```python
from build123d import *

# Parameters (mm, degrees)
BOSS_EXTRUDE2_DEPTH   = 22
SKETCH6_R             = 6
BOSS_EXTRUDE3_DEPTH   = 8
BOSS_EXTRUDE4_DEPTH   = 65
SKETCH8_R             = 3
CUT_EXTRUDE5_DEPTH    = 65
SKETCH9_R             = 6
CUT_EXTRUDE6_DEPTH    = 52
M4_TAPPED_HOLE1_D     = 3.3
M4_TAPPED_HOLE1_DEPTH = 14
M4_TAPPED_HOLE1_TIP   = 0.991420021
SKETCH13_R            = 1.5
SKETCH13_R_2          = 2.5
CUT_EXTRUDE7_DEPTH    = 5
SKETCH14_R            = 1
CUT_EXTRUDE8_DEPTH    = 15
CHAMFER1_SIZE         = 1


with BuildPart() as part:
    # Sketch2 → Boss-Extrude2 (new body)
    with BuildSketch(Plane(origin=(0, 0, 0), x_dir=(1, 0, 0), z_dir=(0, 1, 0))):
        with BuildLine():
            Line((3.31662479, -5), (-3.31662479, -5))
            ThreePointArc((-3.31662479, -5), (0, 6), (3.31662479, -5))
        make_face()
    extrude(amount=BOSS_EXTRUDE2_DEPTH)

    # Sketch6 → Boss-Extrude3 (add)
    with BuildSketch(Plane(origin=(0, 22, 0), x_dir=(1, 0, 0), z_dir=(0, 1, 0))):
        with Locations(Location((0, 0, 0), (0, 0, 236.442690238))):
            Circle(SKETCH6_R)
    extrude(amount=BOSS_EXTRUDE3_DEPTH)

    # Sketch7 → Boss-Extrude4 (add)
    with BuildSketch(Plane(origin=(0, 30, 0), x_dir=(1, 0, 0), z_dir=(0, 1, 0))):
        with BuildLine():
            Line((-13, 5.196152423), (-13, -5.196152423))
            ThreePointArc((-13, -5.196152423), (14, 0), (-13, 5.196152423))
        make_face()
    extrude(amount=BOSS_EXTRUDE4_DEPTH)

    # Sketch8 → Cut-Extrude5 (cut)
    with BuildSketch(Plane(origin=(0, 95, 0), x_dir=(1, 0, 0), z_dir=(0, 1, 0))):
        with Locations(Location((-8, 0, 0), (0, 0, 270))):
            Circle(SKETCH8_R)
    extrude(amount=-CUT_EXTRUDE5_DEPTH, mode=Mode.SUBTRACT)

    # Sketch9 → Cut-Extrude6 (cut)
    with BuildSketch(Plane(origin=(0, 95, 0), x_dir=(1, 0, 0), z_dir=(0, 1, 0))):
        with Locations(Location((5, 0, 0), (0, 0, 270))):
            Circle(SKETCH9_R)
    extrude(amount=-CUT_EXTRUDE6_DEPTH, mode=Mode.SUBTRACT)

    # M4 Tapped Hole1
    with Locations(Plane(origin=(0, 95, -9), x_dir=(0, 0, 1), z_dir=(0, 1, 0))):
        with Locations((0, 0), (18, 0)):
            Hole(M4_TAPPED_HOLE1_D / 2, depth=M4_TAPPED_HOLE1_DEPTH)
            with Locations((0, 0, -(M4_TAPPED_HOLE1_DEPTH + M4_TAPPED_HOLE1_TIP / 2))):  # 118° drill point
                Cone(0, M4_TAPPED_HOLE1_D / 2, M4_TAPPED_HOLE1_TIP, mode=Mode.SUBTRACT)

    # Sketch13 → Cut-Extrude7 (cut)
    with BuildSketch(Plane.ZY.offset(13)):
        with Locations((0, 34)):
            Circle(SKETCH13_R)
        with Locations((0, 63)):
            Circle(SKETCH13_R_2)
    extrude(amount=-CUT_EXTRUDE7_DEPTH, mode=Mode.SUBTRACT)

    # Sketch14 → Cut-Extrude8 (cut)
    with BuildSketch(Plane.ZY.offset(13)):
        with Locations((0, 85)):
            Circle(SKETCH14_R)
        with Locations((0, 43)):
            Circle(SKETCH14_R)
    extrude(amount=-CUT_EXTRUDE8_DEPTH, mode=Mode.SUBTRACT)

    # Chamfer1
    chamfer1_edges = [part.edges().sort_by_distance(p)[0] for p in [
        (0, 0, 5),
        (0, 0, -6),
    ]]
    chamfer(chamfer1_edges, length=CHAMFER1_SIZE - 0.0001)  # a hair under: the kernel refuses the full size


solid = part.part
```
Model file for the job. Use its own axes, mm. A direction names the side the tool comes from. Coordinates: 2 decimals unless noted, no trailing zeros. Order: outer loops, then holes, each group sorted by start corner. A loop starts at its lowest first (then second) coordinate and runs counter-clockwise, first axis right, second up. Notation, with made-up numbers: (-35.5, 28) - (11.5, 28) arc R7 ccw to (11.5, 39) - close; hole circle Ø5 at (-35.5, 56). An arc over 180 degrees is marked (long way). Return JSON: item names as keys, results as strings. Group by question number.
1) Flat gauge pins, fed straight in: P1, Ø1.2, axis at y = 85, z = 0, coming from the -X side; P2, Ø1.5, axis at y = 31.5, z = -1, coming from the +X side; P3, Ø1.5, axis at x = -6.5, y = 67.5, coming from the -Z side. Where does each tip first touch, or does it go through?
2) Tool access for faces 4 (the flat face through (-13, 62, -4)), 5 (the cylindrical face through (-3, 84, 0)), 6 (the cylindrical face through (0.07, 87.9, 10.65)): list every direction of +Z, -Z, +X, -X, +Y, -Y with a clear straight run to the whole face (end or side of a thin tool).
3) Mould opens along Y. For faces 1 (the cylindrical face through (6.802, 69.364, 5.723)), 2 (the cylindrical face through (-11.82, 34.45, 1.43)), 3 (the conical face through (-0.1, 80.2, -8.7)) say: released by +Y, released by -Y, zero draft, split by the parting line, or undercut.
4) Saw through at C-C, the plane y = 34. Write the cut outline in (x, z), plus the area to 3 significant figures.
5) Probe line 1 (Y direction, x = -11.85, z = 0); line 2 (Y direction, x = -4.05, z = 0); line 3 (Z direction, x = 0, y = 85). List the from-to ranges inside material, lowest first. Write a range as from..to.
6) Saw through at D-D, the plane x = 7.75. Write the cut outline in (y, z), plus the area to 3 significant figures.
7) Saw through at B-B, the plane z = 0. Count the separate pieces of the cut face and the enclosed holes in it, plus the area to 3 significant figures.
8) Saw through at A-A, the plane y = 85. Write the cut outline in (x, z).
Values found:
{
 "1": {"P1": "stops at x = 10.97", "P2": "stops at x = 14", "P3": "stops at z = -12.76"},
 "2": {"face 4": "+Z, -Z, -X, +Y, -Y", "face 5": "-X", "face 6": "+Y"},
 "3": {"face 1": "zero draft", "face 2": "undercut", "face 3": "released by +Y"},
 "4": {"outline": "(-13, -5.2) arc R14 ccw (long way) to (-13, 5.2) - (-13, 1.5) - (-10.6, 1.5) arc R3 cw (long way) to (-10.6, -1.5) - (-13, -1.5) - close", "area": "574 mm²"},
 "5": {"line 1": "y = 30..32.5, 35.5..42, 44..60.5, 65.5..84, 86..95", "line 2": "y = 0..42, 44..84, 86..95", "line 3": "z = -14..-10.65, -7.35..-3.32, 3.32..7.35, 10.65..14"},
 "6": {"outline": "(30, -11.66) - (95, -11.66) - (95, -5.33) - (43, -5.33) - (43, 5.33) - (95, 5.33) - (95, 11.66) - (30, 11.66) - close", "area": "961 mm²"},
 "7": {"separate pieces": "8", "enclosed holes": "0", "area": "1,060 mm²"},
 "8": {"outline": "(-13, -5.2) arc R14 ccw (long way) to (-13, 5.2) - (-13, 1) - (-10.83, 1) arc R3 cw to (-5.17, 1) - (-0.92, 1) arc R6 cw (long way) to (-0.92, -1) - (-5.17, -1) arc R3 cw to (-10.83, -1) - (-13, -1) - close; hole circle Ø3.3 at (0, -9); hole circle Ø3.3 at (0, 9)"}
}
